Can you work these out from the model? Positions are in its coordinate system, mm. Coordinates: 2 decimals unless noted, no trailing zeros. Loops run counter-clockwise (first coordinate to the right, second up) from the corner with the lowest first, then second, coordinate; pieces in that order, holes last.
```python
from build123d import *

# Parameters (mm, degrees)
SKETCH1_W           = 240
SKETCH1_H           = 974
SKETCH1_W_2         = 120
SKETCH1_H_2         = 183
BOSS_EXTRUDE1_DEPTH = 10
MOVE_FACE1_BY       = 5
MOVE_FACE2_BY       = 105


with BuildPart() as part:
    # Sketch1 → Boss-Extrude1 (new body)
    with BuildSketch(Plane.XY):
        with Locations((120, 487)):
            Rectangle(SKETCH1_W, SKETCH1_H)
        with Locations((170, 128.5)):
            Rectangle(SKETCH1_W_2, SKETCH1_H_2, mode=Mode.SUBTRACT)
        with Locations((170, 356.5)):
            Rectangle(SKETCH1_W_2, SKETCH1_H_2, mode=Mode.SUBTRACT)
        with Locations((170, 584.5)):
            Rectangle(SKETCH1_W_2, SKETCH1_H_2, mode=Mode.SUBTRACT)
        with Locations((170, 812.5)):
            Rectangle(SKETCH1_W_2, SKETCH1_H_2, mode=Mode.SUBTRACT)
    extrude(amount=BOSS_EXTRUDE1_DEPTH)

    # Move Face1: a face moved outward by 5.0
    extrude(part.faces().sort_by_distance((0, 487, 5))[0], amount=MOVE_FACE1_BY, dir=(-1, 0, 0))

    # Move Face2: a face moved outward by 105.0
    extrude(part.faces().sort_by_distance((240, 487, 5))[0], amount=MOVE_FACE2_BY, dir=(1, 0, 0))


solid = part.part
```
(1) I want a section at A-A on y = 643.5. Write out the boundary of the cut face in (x, z), then the cut area to 3 significant figures.
Check values:
outline: (-5, 0) - (110, 0) - (110, 10) - (-5, 10) - close; (230, 0) - (345, 0) - (345, 10) - (230, 10) - close
area: 2,300 mm2
(2) I want a section at C-C on z = 6. Write out the boundary of the cut face in (x, y).
Check values:
outline: (-5, 0) - (345, 0) - (345, 974) - (-5, 974) - close; hole (110, 37) - (230, 37) - (230, 220) - (110, 220) - close; hole (110, 265) - (230, 265) - (230, 448) - (110, 448) - close; hole (110, 493) - (230, 493) - (230, 676) - (110, 676) - close; hole (110, 721) - (230, 721) - (230, 904) - (110, 904) - close
(3) I want a section at B-B on x = 215. Write out the boundary of the cut face in (y, z), then the cut area to 3 significant figures.
Check values:
outline: (0, 0) - (37, 0) - (37, 10) - (0, 10) - close; (220, 0) - (265, 0) - (265, 10) - (220, 10) - close; (448, 0) - (493, 0) - (493, 10) - (448, 10) - close; (676, 0) - (721, 0) - (721, 10) - (676, 10) - close; (904, 0) - (974, 0) - (974, 10) - (904, 10) - close
area: 2,420 mm2
(4) If I drill on probe 1 along Y at (x, z) = (126, 9.25); probe 2 along X at (y, z) = (341.5, 0.75), over which ranges is the centre line in solid material (lowest first)?
Check values:
probe 1: y = 0 to 37, 220 to 265, 448 to 493, 676 to 721, 904 to 974
probe 2: x = -5 to 110, 230 to 345
